from build123d import *

# Parameters (mm, degrees)
SKETCH_1_W          = 500
SKETCH_1_H          = 40
EXTRUDE_1_DEPTH     = 4
SKETCH_3_W          = 40
SKETCH_3_H          = 30
CUT_EXTRUDE_1_DEPTH = 502.61339695
SKETCH_4_W          = 40
SKETCH_4_H          = 30
CUT_EXTRUDE_2_DEPTH = 502.61339695


with BuildPart() as part:
    # Эскиз1 → Бобышка-Вытянуть1 (new body)
    with BuildSketch(Plane(origin=(0, 0, 0), x_dir=(1, 0, 0), z_dir=(0, 1, 0))):
        with Locations((250, 20)):
            Rectangle(SKETCH_1_W, SKETCH_1_H)
    extrude(amount=EXTRUDE_1_DEPTH)

    # Эскиз3 → Вырез-Вытянуть1 (cut, through all)
    with BuildSketch(Plane(origin=(0, 4, 0), x_dir=(1, 0, 0), z_dir=(0, 1, 0))):
        with Locations((20, 25)):
            Rectangle(SKETCH_3_W, SKETCH_3_H)
    extrude(amount=-CUT_EXTRUDE_1_DEPTH, mode=Mode.SUBTRACT)

    # Эскиз4 → Вырез-Вытянуть2 (cut, through all)
    with BuildSketch(Plane(origin=(0, 4, 0), x_dir=(1, 0, 0), z_dir=(0, 1, 0))):
        with Locations((480, 25)):
            Rectangle(SKETCH_4_W, SKETCH_4_H)
    extrude(amount=-CUT_EXTRUDE_2_DEPTH, mode=Mode.SUBTRACT)


solid = part.part
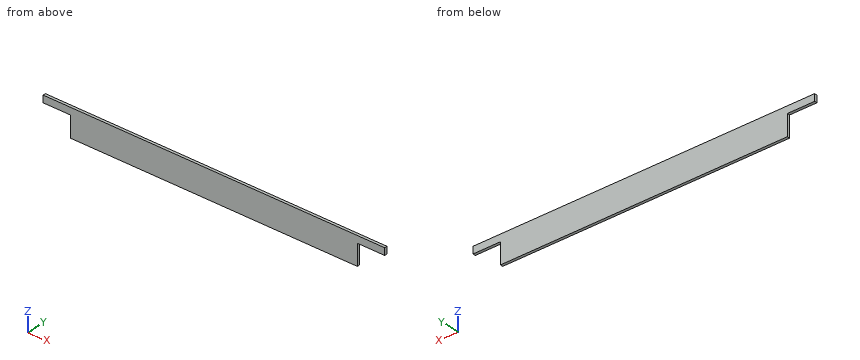
The listing builds one solid part. Answer for the finished solid, in the listing's coordinates (mm). Round coordinates to 2 decimals unless told otherwise and drop trailing zeros. Order: outer loops, then holes, each group sorted by start corner. A loop starts at its lowest first (then second) coordinate and runs counter-clockwise, first axis right, second up. Notation, with made-up numbers: (-29.5, 87) -> (10.5, 87) arc R28 ccw to (10.5, 111) -> close; hole circle Ø10 at (48, -37). An arc over 180 degrees is marked (long way). Write each question's results on one line, items separated by ' | '. Start each with the question number.
Q1. A straight line is drawn through the part: probe 1 along X at (y, z) = (2.15, -21). Find the intervals that lie inside material, in ascending order. Write a range as from..to.
Q2. Find section B-B (z = -16). Determine the outline of the cut face in (x, y), then the cut area to 3 significant figures.
Q3. Each of these flat-tipped pins is pushed along its axis until it touches: pin 1 (2 mm diameter, centred on x = 28, y = 3, fed in from -Z); pin 2 (1.2 mm diameter, centred on y = 1.5, z = -25, fed in from +X). Where does it stop, or does it pass through?
Q4. Find section A-A (y = 1.7). Determine the outline of the cut face in (x, z).
Worked answers:
1) probe 1: x = 40..460
2) outline: (40, 0) -> (460, 0) -> (460, 4) -> (40, 4) -> close | area: 1,680 mm2
3) pin 1: stops at z = -10 | pin 2: stops at x = 460
4) outline: (0, -10) -> (40, -10) -> (40, -40) -> (460, -40) -> (460, -10) -> (500, -10) -> (500, 0) -> (0, 0) -> close
